Source: CAD feature listing. Evaluate the final solid. Frame: model axes, mm. A direction names the side the tool comes from. Coordinates: 2 decimals unless noted, no trailing zeros. Loops run counter-clockwise (first coordinate to the right, second up) from the corner with the lowest first, then second, coordinate; pieces in that order, holes last.
Autodesk Inventor part; units mm, degrees
ref_plane "YZ Plane" through (0, 0, 0) normal (1, 0, 0) x (0, 1, 0)
ref_plane "XZ Plane" through (0, 0, 0) normal (0, 1, 0) x (-1, 0, 0)
ref_plane "XY Plane" through (0, 0, 0) normal (0, 0, 1) x (1, 0, 0)
sketch "Sketch1" plane through (0, 0, 0) normal (0, 1, 0) x (-1, 0, 0)
  line L0 (0, 0) -> (20.32, 0)
  line L1 (20.32, 0) -> (20.32, -88.9)
  line L2 (20.32, -88.9) -> (0, -88.9)
  line L3 (0, -88.9) -> (0, 0)
  line L4 (10.16, -88.9) -> (10.16, -74.93) construction
  circle A0 centre (10.16, -74.93) radius 2.3368
  circle A1 centre (10.16, -11.43) radius 2.3368
  dimension "d0" = 20.32
  dimension "d1" = 88.9
  dimension "d2" = 13.97
  dimension "d3" = 4.6736
  dimension "d4" = 63.5
extrude "Extrusion1" add sketch "Sketch1" along normal blind 37.084
sketch "Sketch2" plane through (0, 37.084, 0) normal (0, 1, 0) x (1, 0, 0)
  line L0 (-60.96, 60.325) -> (40.64, 60.325)
  line L1 (40.64, 60.325) -> (40.64, 28.575)
  line L2 (40.64, 28.575) -> (-60.96, 28.575)
  line L3 (-60.96, 28.575) -> (-60.96, 60.325)
  line L4 (0, 88.9) -> (-20.32, 88.9)
  line L5 (-10.16, 60.325) -> (-10.16, 28.575)
  line L6 (-60.96, 44.45) -> (40.64, 44.45) construction
  circle A0 centre (-48.26, 44.45) radius 2.3368
  circle A1 centre (27.94, 44.45) radius 2.3368
  circle A2 centre (-10.16, 74.93) radius 2.3368
  line L7 (-10.16, 88.9) -> (-10.16, 44.45)
  point P0 (0, 0)
  point P1 (-12.351, 76.2)
  point P2 (-15.843, 76.2)
  dimension "d8" = 31.75
  dimension "d9" = 101.6
  dimension "d11" = 4.6736
  dimension "d17" = 44.45
  dimension "d18" = 38.1
  dimension "d19" = 38.1
extrude "Extrusion2" add sketch "Sketch2" against normal blind 3.175 contours L0 L5 L2 L3 | L0 L1 L2 L5
sketch "Sketch3" plane through (0, 37.084, 0) normal (0, 1, 0) x (1, 0, 0)
  circle A0 centre (-10.16, 11.43) radius 2.3368
  circle A1 centre (-10.16, 11.43) radius 4.445
  circle A2 centre (-10.16, 74.93) radius 2.3368
  circle A3 centre (-10.16, 74.93) radius 4.445
  point P0 (0, 0)
  dimension "d20" = 8.89
extrude "Extrusion3" cut sketch "Sketch3" against normal blind 16.002 contours A0 | A1 | A2 | A3
fillet "Fillet1" radius 6.35 4 edges at (-20.32, 18.542, -88.9) (0, 18.542, -88.9) (-20.32, 18.542, 0) (0, 18.542, 0)
fillet "Fillet2" radius 6.35 8 edges at (-60.96, 35.4965, -60.325) (-60.96, 35.4965, -28.575) (-20.32, 35.4965, -28.575) (0, 35.4965, -28.575) (40.64, 35.4965, -28.575) (40.64, 35.4965, -60.325) (0, 35.4965, -60.325) (-20.32, 35.4965, -60.325)
fillet "Fillet3" radius 6.35 2 edges at (-20.32, 33.909, -44.45) (0, 33.909, -44.45)
sketch "Sketch4" plane through (0, 37.084, 0) normal (0, 1, 0) x (1, 0, 0)
  line L0 (-6.35, 88.9) -> (-13.97, 88.9)
  line L1 (-10.16, 88.9) -> (-10.16, 0)
  line L2 (-13.97, 0) -> (-6.35, 0)
  circle A0 centre (-10.16, 74.93) radius 2.3368
  line L3 (-10.16, 80.1878) -> (-5.6066, 77.5589)
  line L4 (-5.6066, 77.5589) -> (-5.6066, 72.3011)
  line L5 (-5.6066, 72.3011) -> (-10.16, 69.6722)
  line L6 (-10.16, 69.6722) -> (-14.7134, 72.3011)
  line L7 (-14.7134, 72.3011) -> (-14.7134, 77.5589)
  line L8 (-14.7134, 77.5589) -> (-10.16, 80.1878)
  circle A1 centre (-10.16, 11.43) radius 2.3368
  line L9 (-10.16, 16.6878) -> (-5.6066, 14.0589)
  line L10 (-5.6066, 14.0589) -> (-5.6066, 8.8011)
  line L11 (-5.6066, 8.8011) -> (-10.16, 6.1722)
  line L12 (-10.16, 6.1722) -> (-14.7134, 8.8011)
  line L13 (-14.7134, 8.8011) -> (-14.7134, 14.0589)
  line L14 (-14.7134, 14.0589) -> (-10.16, 16.6878)
  point P0 (0, 0)
  dimension "d26" = 5.2578
  dimension "d27" = 5.2578
extrude "Extrusion4" cut sketch "Sketch4" against normal up to surface (16.002 mm away) contours L9 L10 L11 L1 A1 | L1 A1 L12 L13 L14 | L6 L7 L8 L1 A0 | L1 A0 L3 L4 L5
properties part number "BRAIN_MOUNT"
Q1. Section query A-A on y = 25. Return the cut outline in (x, z).
Q2. Section query C-C on x = 27.94. Return the cut outline in (y, z) (3 decimals).
Q3. Material intervals for line 1 along Z through (x, y) = (-10.16, 14); line 2 along Z through (x, y) = (-48.26, 36.4) (3 decimals); line 3 along X through (y, z) = (8, -11.5), sorted ascending.
Q4. First-contact query: pin 1 Ø1 at (x, y) = (-16, 17) entering from +Z; pin 2 Ø4 at (y, z) = (31.5, -12.5) entering from +X; pin 3 Ø1.6 at (x, y) = (26, 35.5) entering from -Z (3 decimals); pin 4 Ø4 at (x, z) = (-10.16, -11.43) entering from +Y. Flat tips, straight axial feed; report the tip coordinate or a pass-through.
Q5. Section query D-D on z = -74.93. Return the cut outline in (x, y).
Q6. Draft query along Z for faces 4 (the flat face through (-44, 33.909, -45)), 5 (the cylindrical face through (38.73, 35.474, -58.514)), 6 (the flat face through (-12.405, 29.195, -7.468)), 7 (the flat face through (-10, 18, 0)). Return one class per face: released by +Z, released by -Z, zero draft, split by the parting line, or undercut.
Q7. Section query B-B on z = -44.45. Return the cut outline in (x, y).
Q8. Reachability of faces 1 (the flat face through (-40, 36, -28.575)), 2 (the flat face through (-12.405, 29.195, -70.968)), 3 (the flat face through (21, 36, -28.575)) from +Z, -Z, +X, -X, +Y, -Y: full face, straight path, thin tool, end or side. Return the list, or none.
Resolved:
1. outline: (-20.32, -82.55) arc R6.35 ccw to (-13.97, -88.9) - (-6.35, -88.9) arc R6.35 ccw to (0, -82.55) - (0, -6.35) arc R6.35 ccw to (-6.35, 0) - (-13.97, 0) arc R6.35 ccw to (-20.32, -6.35) - close; hole (-14.71, -77.56) - (-10.16, -80.19) - (-5.61, -77.56) - (-5.61, -72.3) - (-10.16, -69.67) - (-14.71, -72.3) - close; hole (-14.71, -14.06) - (-10.16, -16.69) - (-5.61, -14.06) - (-5.61, -8.8) - (-10.16, -6.17) - (-14.71, -8.8) - close
2. outline: (33.909, -60.325) - (37.084, -60.325) - (37.084, -46.787) - (33.909, -46.787) - close; (33.909, -42.113) - (37.084, -42.113) - (37.084, -28.575) - (33.909, -28.575) - close
3. line 1: z = -88.9 to -77.27, -72.59 to -13.77, -9.09 to 0
3. line 2: z = -60.325 to -46.787, -42.113 to -28.575
3. line 3: x = -20.32 to -12.5, -7.82 to 0
4. pin 1: stops at z = -0.19
4. pin 2: stops at x = 0
4. pin 3: stops at z = -60.325
4. pin 4: passes through
5. outline: (-20.32, 0) - (-12.5, 0) - (-12.5, 21.08) - (-14.71, 21.08) - (-14.71, 37.08) - (-20.32, 37.08) - close; (-7.82, 0) - (0, 0) - (0, 37.08) - (-5.61, 37.08) - (-5.61, 21.08) - (-7.82, 21.08) - close
6. face 4: zero draft
6. face 5: released by -Z
6. face 6: undercut
6. face 7: released by +Z
7. outline: (-60.96, 33.91) - (-50.6, 33.91) - (-50.6, 37.08) - (-60.96, 37.08) - close; (-45.92, 33.91) - (-26.67, 33.91) arc R6.35 cw to (-20.32, 27.56) - (-20.32, 0) - (0, 0) - (0, 27.56) arc R6.35 cw to (6.35, 33.91) - (25.6, 33.91) - (25.6, 37.08) - (-45.92, 37.08) - close; (30.28, 33.91) - (40.64, 33.91) - (40.64, 37.08) - (30.28, 37.08) - close
8. face 1: +Z, -X, +Y, -Y
8. face 2: +Y
8. face 3: +Z, +X, +Y, -Y
